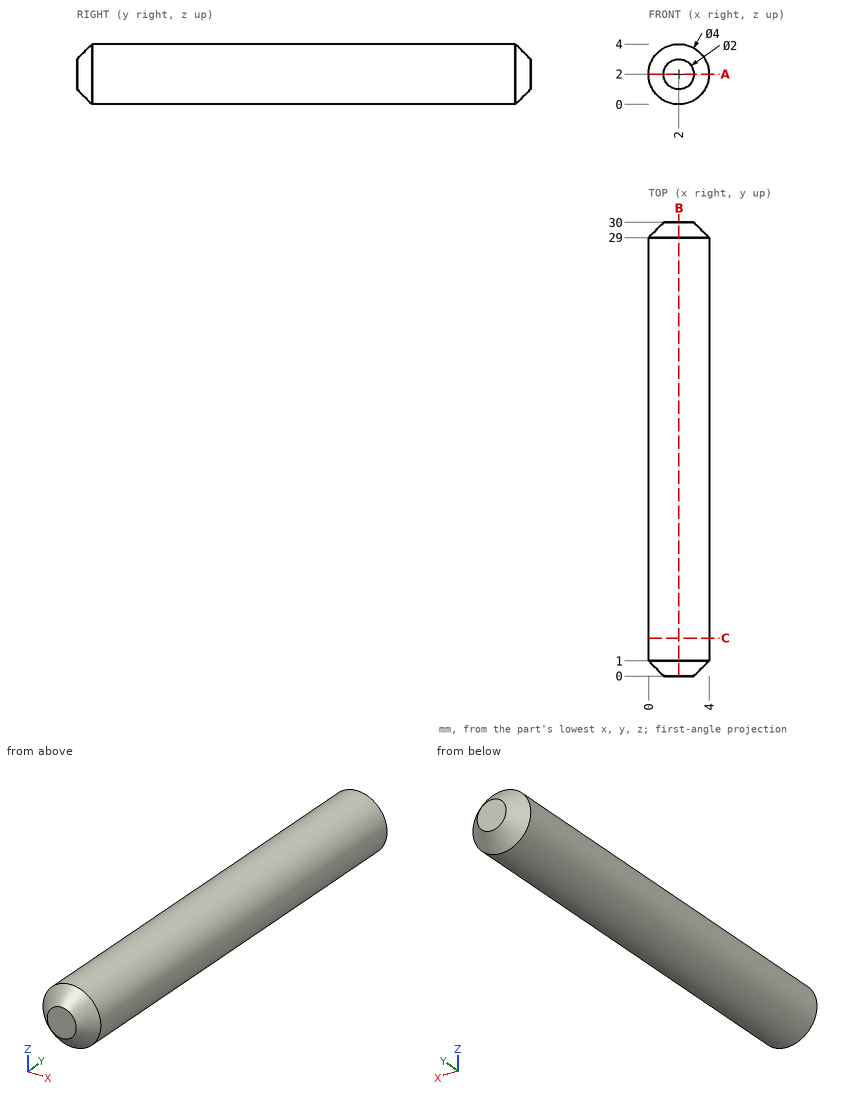
Design review of the part shown in the three views and the two pictorial views. Dimensions are in mm from the part's minimum x, y and z. Round coordinates to 2 decimals unless told otherwise and drop trailing zeros. Loops run counter-clockwise (first coordinate to the right, second up) from the corner with the lowest first, then second, coordinate; pieces in that order, holes last. Notation, with made-up numbers: (-22.75, -17) - (31.25, -17) arc R13 cw to (31.25, 8) - close; hole circle Ø3 at (68, 41.5). An arc over 180 degrees is marked (long way). Answer as CSV lines item,"result".
(1) Consider section C-C on y = 2.5. Give the boundary of the cut face in (x, z), then the cut area to 3 significant figures.
Checked values:
outline,"circle Ø4 at (2, 2)"
area,"12.6 mm2"
(2) Consider section B-B on x = 2. Give the boundary of the cut face in (y, z).
Checked values:
outline,"(0, 1) - (1, 0) - (29, 0) - (30, 1) - (30, 3) - (29, 4) - (1, 4) - (0, 3) - close"
(3) Consider section A-A on z = 2. Give the boundary of the cut face in (x, y), then the cut area to 3 significant figures.
Checked values:
outline,"(0, 1) - (1, 0) - (3, 0) - (4, 1) - (4, 29) - (3, 30) - (1, 30) - (0, 29) - close"
area,"118 mm2"
(4) Wall thickness on line 1 (X direction, y = 5, z = 2.15); line 2 (X direction, y = 17.25, z = 1.3); line 3 (Z direction, x = 0.55, y = 10.25): over which ranges is each line inside the solid? List them lowest first.
Checked values:
line 1,"x = 0.01 to 3.99"
line 2,"x = 0.13 to 3.87"
line 3,"z = 0.62 to 3.38"
